```python
from build123d import *

# Parameters (mm, degrees)
F0_W     = 1193.8
F0_H     = 349.25
F1_DEPTH = 19.3548
F2_W     = 1193.8
F2_H     = 57.15
F3_DEPTH = 17.0942
F5_D     = 6.35


with BuildPart() as f1:
    # F0 (on Top) → F1 (new body)
    with BuildSketch(Plane.XY):
        Rectangle(F0_W, F0_H)
    extrude(amount=F1_DEPTH)

    # F2 (on face) → F3 (join)
    with BuildSketch(Plane(origin=(0, 0, 0), x_dir=(1, 0, 0), z_dir=(0, 0, -1))):
        Rectangle(F2_W, F2_H)
    extrude(amount=F3_DEPTH)

    # F5 (through all)
    with Locations(Plane(origin=(-596.9, 0, 0), x_dir=(0, -1, 0), z_dir=(-1, 0, 0))):
        with Locations((-21.59, -8.5471), (21.59, -8.5471)):
            Hole(F5_D / 2)


solid = f1.part
```
The listing builds one solid part. Answer for the finished solid, in the listing's coordinates (mm). A direction names the side the tool comes from. Coordinates: 2 decimals unless noted, no trailing zeros. Write each loop counter-clockwise with the first axis right and the second up, starting at its lowest first coordinate (ties: lowest second). Pieces come first, ordered by that corner, then holes. Notation, with made-up numbers: (53, 12) - (64, 12) arc R15 cw to (64, 28) - close; hole circle Ø6 at (-32.5, 18). An arc over 180 degrees is marked (long way). Return JSON: item names as keys, results as strings. Group by question number.
Q1. Which of the six approach directions +Z, -Z, +X, -X, +Y, -Y give full straight-line access (tool end or side, diameter ignored) to faces 1 (the flat face through (-8, -174.625, 10)), 2 (the flat face through (-8, -101, 0)), 3 (the flat face through (-8, 103, 0))?
Q2. Find the intervals of material crossed by line 1 along Z through (x, y) = (270, 21.59); line 2 along Y through (x, z) = (-316, -9.5) (3 decimals); line 3 along Y through (x, z) = (74, -11) (3 decimals), in increasing order. Write a range as [from, to].
Q3. The part is cut by section A-A on x = 178.5. Write down the section's boundary in (y, z) (3 decimals).
Q4. The part is cut by section B-B on y = 142.5. Write down the section's boundary in (x, z).
Q5. Flat-ended cylindrical pins translate along their axes: pin 1 Ø5 at (x, z) = (265.5, -8.5) entering from -Y (3 decimals); pin 2 Ø7.5 at (y, z) = (-21.59, -8.55) entering from +X; pin 3 Ø4 at (x, y) = (13.5, 139.5) entering from -Z; pin 4 Ø19 at (x, z) = (-204.5, -11) entering from +Y (3 decimals). Find the tip coordinate at first contact, or state that the pin passes through.
Evaluation:
{
 "1": {"face 1": "+Z, -Z, +X, -X, -Y", "face 2": "-Z, +X, -X, -Y", "face 3": "-Z, +X, -X, +Y"},
 "2": {"line 1": "z = [-17.09, -11.72], [-5.37, 19.35]", "line 2": "y = [-28.575, -24.619], [-18.561, 18.561], [24.619, 28.575]", "line 3": "y = [-28.575, -23.606], [-19.574, 19.574], [23.606, 28.575]"},
 "3": {"outline": "(-174.625, 0) - (-28.575, 0) - (-28.575, -17.094) - (28.575, -17.094) - (28.575, 0) - (174.625, 0) - (174.625, 19.355) - (-174.625, 19.355) - close; hole circle Ø6.35 at (-21.59, -8.547); hole circle Ø6.35 at (21.59, -8.547)"},
 "4": {"outline": "(-596.9, 0) - (596.9, 0) - (596.9, 19.35) - (-596.9, 19.35) - close"},
 "5": {"pin 1": "stops at y = -28.575", "pin 2": "stops at x = 596.9", "pin 3": "stops at z = 0", "pin 4": "stops at y = 28.575"}
}
